Can you work these out from the model? Positions are in its coordinate system, mm. Round coordinates to 2 decimals unless told otherwise and drop trailing zeros. Order: outer loops, then holes, each group sorted by start corner. A loop starts at its lowest first (then second) coordinate and runs counter-clockwise, first axis right, second up. Notation, with made-up numbers: M 2.25,-9 L 20.25,-9 A16 cw 20.25,16 Z; hole C 68.5,-2 d1. An arc over 180 degrees is marked long. Answer as a JSON object with one key per item and string values. Group by question number.
from build123d import *

# Parameters (mm, degrees)
SKETCH1_R           = 12.1
SKETCH1_R_2         = 10.6
BOSS_EXTRUDE1_DEPTH = 100
SKETCH8_R           = 2
CUT_EXTRUDE2_DEPTH  = 104.616567834


with BuildPart() as part:
    # Sketch1 → Boss-Extrude1 (new body)
    with BuildSketch(Plane.XY):
        with Locations((0.713024601, 11.821110558)):
            Circle(SKETCH1_R)
        with Locations((0.713024601, 11.821110558)):
            Circle(SKETCH1_R_2, mode=Mode.SUBTRACT)
    boss_extrude1 = extrude(amount=BOSS_EXTRUDE1_DEPTH)

    # Sketch8 → Cut-Extrude2 (cut, symmetric)
    with BuildSketch(Plane(origin=(0, 0, 0), x_dir=(0, 0, -1), z_dir=(1, 0, 0))):
        with Locations((-84.375, 12.221110558)):
            Circle(SKETCH8_R)
        with Locations((-151.625, 12.221110558)):
            Circle(SKETCH8_R)
    cut_extrude2 = extrude(amount=CUT_EXTRUDE2_DEPTH, both=True, mode=Mode.SUBTRACT)

    # Mirror1: Boss-Extrude1, Cut-Extrude2 across plane
    add(boss_extrude1.mirror(Plane(origin=(0.713024601, 11.821110558, 0), x_dir=(1, 0, 0), z_dir=(0, 0, 1))))
    add(cut_extrude2.mirror(Plane(origin=(0.713024601, 11.821110558, 0), x_dir=(1, 0, 0), z_dir=(0, 0, 1))), mode=Mode.SUBTRACT)


solid = part.part
Item 1: If we mould it in two halves opening along Z, with no side actions, what happens to faces 1 (the face through (1, 1, 100)), 2 (the face through (1, 1, -100)), 3 (the face through (-10.488, 11.455, 82.528))? For each: +Z half, -Z half, draft (parallel to the pull), parting line (faces both ways), or undercut.
Item 2: Suppose I cut it at C-C, the plane z = -68. Write out the boundary of the cut face in (x, y).
Item 3: I need wall thicknesses on line 1 (Y direction, x = 0.25, z = -70); line 2 (X direction, y = 12.5, z = -88); line 3 (Z direction, x = -10, y = 11.25). Which ranges of each line are inside material? Lowest first, please.
Item 4: I'm going to push flat-ended pins straight in: pin 1 Ø1.5 at (y, z) = (17, -54) entering from +X; pin 2 Ø10 at (x, z) = (9, -30.5) entering from -Y; pin 3 Ø1 at (x, z) = (-9, -59.5) entering from -Y; pin 4 Ø1 at (x, y) = (9, 12.5) entering from +Z. Where does each tip first touch, or does it pass through?
Item 5: Suppose I cut it at B-B, the plane x = -7.75. Write out the boundary of the cut face in (y, z), and give its area (3 significant figures).
Item 6: Suppose I cut it at A-A, the plane y = 8.25. Write out the boundary of the cut face in (x, z).
Computed:
{
 "1": {"face 1": "+Z half", "face 2": "-Z half", "face 3": "undercut"},
 "2": {"outline": "C 0.71,11.82 d24.2; hole C 0.71,11.82 d21.2"},
 "3": {"line 1": "y = -0.27 to 1.23, 22.41 to 23.91", "line 2": "x = -11.37 to -9.87, 11.29 to 12.79", "line 3": "z = -100 to -86.12, -82.63 to 82.63, 86.12 to 100"},
 "4": {"pin 1": "stops at x = 11.97", "pin 2": "stops at y = 0.18", "pin 3": "stops at y = 3.98", "pin 4": "passes through"},
 "5": {"outline": "M 3.17,-100 L 5.44,-100 L 5.44,100 L 3.17,100 Z; M 18.2,-100 L 20.47,-100 L 20.47,100 L 18.2,100 Z", "area": "906 mm^2"},
 "6": {"outline": "M -10.85,-100 L -9.27,-100 L -9.27,100 L -10.85,100 Z; M 10.69,-100 L 12.27,-100 L 12.27,100 L 10.69,100 Z"}
}
